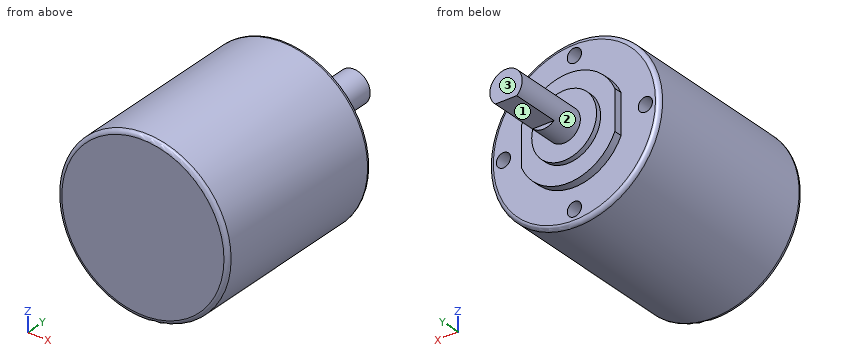
Autodesk Inventor part; units mm, degrees
ref_plane "YZ Plane" through (0, 0, 0) normal (1, 0, 0) x (0, 1, 0)
ref_plane "XZ Plane" through (0, 0, 0) normal (0, 1, 0) x (-1, 0, 0)
ref_plane "XY Plane" through (0, 0, 0) normal (0, 0, 1) x (1, 0, 0)
sketch "スケッチ1" plane through (0, 0, 0) normal (0, 0, 1) x (1, 0, 0)
  line L0 (0, 0) -> (21, 0)
  line L1 (21, 0) -> (21, 45.9)
  line L2 (21, 45.9) -> (12.5, 45.9)
  line L3 (12.5, 45.9) -> (12.5, 47.9)
  line L4 (12.5, 47.9) -> (8, 47.9)
  line L5 (8, 47.9) -> (8, 49.2)
  line L6 (8, 49.2) -> (4, 49.2)
  line L7 (4, 49.2) -> (4, 67.9)
  line L8 (4, 67.9) -> (0, 67.9)
  line L9 (0, 67.9) -> (0, 0)
  dimension "d0" = 21
  dimension "d1" = 4
  dimension "d2" = 12.5
  dimension "d3" = 2
  dimension "d4" = 8
  dimension "d5" = 1.3
  dimension "d6" = 45.9
  dimension "d8" = 20
revolve "回転1" add sketch "スケッチ1" angle 360 about axis through (0, 67.9, 0) along (0, -1, 0)
sketch "スケッチ2" plane through (0, 67.9, 0) normal (0, 1, 0) x (1, 0, 0)
  line L0 (-2.6458, 3) -> (2.6458, 3)
  circle A0 centre (0, 0) radius 4
  arc A1 (2.6458, 3) -> (-2.6458, 3) centre (0, 0) ccw
  dimension "d10" = 3
extrude "押し出し1" cut sketch "スケッチ2" against normal blind 12 contours A0 L0 picked at (0.5822, 3.4764)
sketch "スケッチ4" plane through (0, 47.9, 0) normal (0, 1, 0) x (1, 0, 0)
  line L0 (0, 0) -> (0, 29.0549) construction
  arc A0 (11.5, -4.899) -> (11.5, 4.899) centre (0, 0) ccw
  line L1 (11.5, 4.899) -> (11.5, -4.899)
  circle A1 centre (0, 0) radius 12.5
  arc A2 (-11.5, 4.899) -> (-11.5, -4.899) centre (0, 0) ccw
  line L2 (-11.5, 4.899) -> (-11.5, -4.899)
  dimension "d13" = 11.5
extrude "押し出し2" cut sketch "スケッチ4" against normal blind 2 contours L1 A0 | A1 L2
fillet "フィレット1" radius 1 2 edges at (-21, 45.9, 0) (-21, 0, 0)
sketch "スケッチ5" plane through (0, 45.9, 0) normal (0, 1, 0) x (1, 0, 0)
  circle A0 centre (0, 0) radius 17.5 construction
  circle A1 centre (-17.5, 0) radius 1.75
  line L0 (0, 0) -> (-17.5, 0) construction
  circle A2 centre (0, -17.5) radius 1.75
  circle A3 centre (17.5, 0) radius 1.75
  circle A4 centre (0, 17.5) radius 1.75
  dimension "d18" = 35
  dimension "d17" = 3.5
  dimension "d21" = 360
extrude "押し出し3" cut sketch "スケッチ5" against normal blind 5
properties part number "IG42C-144"
Could you check a few things on this model? Use its own coordinates, in mm. Face numbers are marked on the shaded views. A direction names the side the tool comes from. Give positions to 0.01 mm unless a question says otherwise; leave off trailing zeros. Order: outer loops, then holes, each group sorted by start corner. A loop starts at its lowest first (then second) coordinate and runs counter-clockwise, first axis right, second up. Notation, with made-up numbers: (-24, -0.75) - (-20, -0.75) arc R13 cw to (-20, 9.25) - close; hole circle Ø2 at (-22, -13). An arc over 180 degrees is marked (long way). One line per item, written item: value. Start each with the question number.
1. Imagine slicing it at B-B on y = 50.5. List the corners of the cut face in (x, z) for me, plus the area to 3 significant figures.
2. Imagine slicing it at C-C on y = 20. List the corners of the cut face in (x, z) for me, plus the area to 3 significant figures.
3. Imagine slicing it at A-A on z = 0. List the corners of the cut face in (x, y) for me, plus the area to 3 significant figures.
4. For P1, Ø5.5, axis at x = 0, z = -17.5, coming from the +Y side; P2, Ø1.8, axis at x = 17.5, z = 0, coming from the +Y side; P3, Ø1, axis at x = 11, z = -3.5, coming from the +Y side, each with a flat end and sliding along its axis, tell me the tip position at first contact or that it passes through.
5. Imagine slicing it at D-D on y = 59. List the corners of the cut face in (x, z) for me, plus the area to 3 significant figures.
6. For the marked faces 1, 2 and 3, which set-ups out of +Z, -Z, +X, -X, +Y, -Y let a thin tool reach every point of the face, with its end or its side?
7. If I drill on probe 1 along Z at (x, y) = (0, 44.25); probe 2 along Y at (x, z) = (-6.5, -5); probe 3 along Y at (x, z) = (15.5, -9), over which ranges is the centre line in solid material (lowest first)?
Values:
1. outline: circle Ø8 at (0, 0)
1. area: 50.3 mm²
2. outline: circle Ø42 at (0, 0)
2. area: 1,390 mm²
3. outline: (-21, 1) arc R1 ccw to (-20, 0) - (20, 0) arc R1 ccw to (21, 1) - (21, 44.9) arc R1 ccw to (20, 45.9) - (19.25, 45.9) - (19.25, 40.9) - (15.75, 40.9) - (15.75, 45.9) - (11.5, 45.9) - (11.5, 47.9) - (8, 47.9) - (8, 49.2) - (4, 49.2) - (4, 67.9) - (-4, 67.9) - (-4, 49.2) - (-8, 49.2) - (-8, 47.9) - (-11.5, 47.9) - (-11.5, 45.9) - (-15.75, 45.9) - (-15.75, 40.9) - (-19.25, 40.9) - (-19.25, 45.9) - (-20, 45.9) arc R1 ccw to (-21, 44.9) - close
3. area: 2,110 mm²
4. P1: y = 45.9
4. P2: y = 40.9
4. P3: y = 47.9
5. outline: (-2.65, -3) - (2.65, -3) arc R4 ccw (long way) to start
5. area: 46.6 mm²
6. face 1: -Z, +X, -X, +Y
6. face 2: +Y
6. face 3: +Z, -Z, +X, -X, +Y
7. probe 1: -21 to -19.25, -15.75 to 15.75, 19.25 to 21
7. probe 2: 0 to 47.9
7. probe 3: 0 to 45.9
